Check sheet for the modelled part. Datum: model origin and axes. Units: mm. A direction names the side the tool comes from. Round coordinates to 2 decimals unless told otherwise and drop trailing zeros. Loops run counter-clockwise (first coordinate to the right, second up) from the corner with the lowest first, then second, coordinate; pieces in that order, holes last. Notation, with made-up numbers: (47, -39.75) - (59, -39.75) arc R30 ccw to (59, -15.75) - close; hole circle Ø2 at (18, 19.25). An arc over 180 degrees is marked (long way). Answer in a Markdown table with one row per item. Add a question column.
(1) Cross-section at D-D on z = 44. Enter the section's corners in (x, y).
(2) Access from +Z, -Z, +X, -X, +Y, -Y to the whole of each face (thin tool, end or side, straight path). Record for faces 4 (the cylindrical face through (24.84, -15.21, 12.92)), 5 (the flat face through (23.145, 4.93, -30.382)).
(3) Thickness scan on line 1 along Y through (x, z) = (-7.5, 40); line 2 along Z through (x, y) = (7, -19.5); line 3 along Z through (x, y) = (12, -15.5). Record the ranges inside material, lowest first.
(4) Gauge pin test, flat ends, axial feed: pin 1 (3 mm diameter, centred on x = -10.5, z = -15.5, fed in from -Y); pin 2 (10 mm diameter, centred on x = -5, y = -23.5, fed in from +Z); pin 3 (2 mm diameter, centred on x = -1.5, y = -23.5, fed in from -Z); pin 4 (25 mm diameter, centred on x = 0, z = 0, fed in from +Y). Record the tip position at first contact, or that the pin passes through.
(5) Cross-section at C-C on y = -4. Enter the section's corners in (x, z), then the cut area to 3 significant figures.
(6) Cross-section at B-B on z = 0. Enter the section's corners in (x, y).
(7) Mould release check, pull along X, two halves, no side actions. Record for faces 1 (the cylindrical face through (-29.356, 5.07, -0.177)), 2 (the cylindrical face through (0, 5, 38)), 3 (the cylindrical face through (0, 5, -63)): +X half, -X half, draft (parallel to the pull), parting line (faces both ways), or undercut.
(8) Cross-section at A-A on x = 0. Enter the section's corners in (y, z).
from build123d import *

# Parameters (mm, degrees)
SKETCH1_R           = 14
SKETCH1_R_2         = 19
SKETCH1_R_3         = 6
BOSS_EXTRUDE1_DEPTH = 10
FILLET1_R           = 50


with BuildPart() as part:
    # Sketch1 → Boss-Extrude1 (new body)
    # profile 1 of 3: a face of its own
    with BuildSketch(Plane(origin=(0, 0, 0), x_dir=(1, 0, 0), z_dir=(0, 1, 0))):
        with BuildLine():
            Line((-18.395196505, 48.755706629), (-31, 0))
            Line((-31, 0), (-18.395196505, -48.755706629))
            ThreePointArc((-18.395196505, -48.755706629), (-2.397005048, -25.151807333), (19, -44))
            ThreePointArc((19, -44), (18.848192667, -46.397005048), (18.395196505, -48.755706629))
            Line((18.395196505, -48.755706629), (31, 0))
            Line((31, 0), (18.395196505, 48.755706629))
            ThreePointArc((18.395196505, 48.755706629), (18.848192667, 46.397005048), (19, 44))
            ThreePointArc((19, 44), (-2.397005048, 25.151807333), (-18.395196505, 48.755706629))
        make_face()
        with Locations(Location((0, 0, 0), (0, 0, 270))):
            Circle(SKETCH1_R, mode=Mode.SUBTRACT)
    # profile 2 of 3: a face of its own
    with BuildSketch(Plane(origin=(0, 0, 0), x_dir=(1, 0, 0), z_dir=(0, 1, 0))):
        with Locations((0, -44)):
            Circle(SKETCH1_R_2)
        with Locations(Location((0, -44, 0), (0, 0, 270))):
            Circle(SKETCH1_R_3, mode=Mode.SUBTRACT)
    # profile 3 of 3: a face of its own
    with BuildSketch(Plane(origin=(0, 0, 0), x_dir=(1, 0, 0), z_dir=(0, 1, 0))):
        with Locations((0, 44)):
            Circle(SKETCH1_R_2)
        with Locations(Location((0, 44, 0), (0, 0, 270))):
            Circle(SKETCH1_R_3, mode=Mode.SUBTRACT)
    extrude(amount=BOSS_EXTRUDE1_DEPTH)

    # Fillet1
    fillet1_edges = [part.edges().sort_by_distance(p)[0] for p in [
        (-31, 5, 0),
        (31, 5, 0),
    ]]
    fillet(fillet1_edges, radius=FILLET1_R)

    # Sketch2 → Revolve1 (revolve)
    with BuildSketch(Plane.XY, mode=Mode.PRIVATE) as revolve1_sk:
        Polygon((14, 0), (28, 0), (28, -30), (14, -21.917096231), align=None)
    revolve(revolve1_sk.sketch.rotate(Axis((0, 0, 0), (0, -1, 0)), 90), axis=Axis((0, 0, 0), (0, -1, 0)))


solid = part.part
Answers:
| question | item | result |
|---|---|---|
| 1 | outline | (-19.62, 0) - (-6, 0) - (-6, 10) - (-19.62, 10) - close; (6, 0) - (19.62, 0) - (19.62, 10) - (6, 10) - close |
| 2 | face 4 | -Y |
| 2 | face 5 | -Z, +X, +Y, -Y |
| 3 | line 1 | y = 0 to 10 |
| 3 | line 2 | z = -27.11 to -12.12, 12.12 to 27.11 |
| 3 | line 3 | z = -25.3 to -7.21, 7.21 to 25.3 |
| 4 | pin 1 | stops at y = -25.51 |
| 4 | pin 2 | stops at z = 28 |
| 4 | pin 3 | stops at z = -28 |
| 4 | pin 4 | passes through |
| 5 | outline | circle Ø56 at (0, 0); hole circle Ø28 at (0, 0) |
| 5 | area | 1,850 mm^2 |
| 6 | outline | (-29.36, 0) - (-28, 0) - (-28, -30) - (-14, -21.92) - (-14, 10) - (-29.36, 10) - close; (14, -21.92) - (28, -30) - (28, 0) - (29.36, 0) - (29.36, 10) - (14, 10) - close |
| 7 | face 1 | -X half |
| 7 | face 2 | undercut |
| 7 | face 3 | parting line |
| 8 | outline | (-30, -28) - (0, -28) - (0, -38) - (10, -38) - (10, -14) - (-21.92, -14) - close; (-30, 28) - (-21.92, 14) - (10, 14) - (10, 38) - (0, 38) - (0, 28) - close; (0, -63) - (10, -63) - (10, -50) - (0, -50) - close; (0, 50) - (10, 50) - (10, 63) - (0, 63) - close |
